Autodesk Inventor part; units mm, degrees
ref_plane "YZ Plane" through (0, 0, 0) normal (1, 0, 0) x (0, 1, 0)
ref_plane "XZ Plane" through (0, 0, 0) normal (0, 1, 0) x (-1, 0, 0)
ref_plane "XY Plane" through (0, 0, 0) normal (0, 0, 1) x (1, 0, 0)
sketch "Sketch1" plane through (0, 0, 0) normal (0, 1, 0) x (-1, 0, 0)
  line L0 (3.2, 1.8475) -> (3.2, -1.8475)
  line L1 (3.2, -1.8475) -> (0, -3.695)
  line L2 (0, -3.695) -> (-3.2, -1.8475)
  line L3 (-3.2, -1.8475) -> (-3.2, 1.8475)
  line L4 (-3.2, 1.8475) -> (0, 3.695)
  line L5 (0, 3.695) -> (3.2, 1.8475)
  point P0 (0, 0)
  point P1 (3.2, 0)
  point P2 (-3.2, 0)
  dimension "d0" = 6.4
  dimension "d1" = 120
  dimension "d2" = 6.4
extrude "Extrusion1" add sketch "Sketch1" along normal blind 11.96
sketch "Sketch2" plane through (0, 11.96, 0) normal (0, 1, 0) x (1, 0, 0)
  circle A0 centre (0, 0) radius 1.4224
  dimension "d5" = 2.8448
extrude "Extrusion2" add sketch "Sketch2" along normal blind 4.75
sketch "Sketch3" plane through (0, 0, 0) normal (0, -1, 0) x (1, 0, 0)
  circle A0 centre (0, 0) radius 1.4224
  dimension "d8" = 2.8448
extrude "Extrusion3" cut sketch "Sketch3" against normal blind 6.35
sketch "Sketch4" plane through (0, 0, 0) normal (0, -1, 0) x (1, 0, 0)
  circle A0 centre (0, 0) radius 1.4224
  line L0 (-3.2, -1.8475) -> (-3.2, 1.8475)
  line L1 (0, -3.695) -> (-3.2, -1.8475)
  line L2 (3.2, -1.8475) -> (0, -3.695)
  line L3 (3.2, 1.8475) -> (3.2, -1.8475)
  line L4 (0, 3.695) -> (3.2, 1.8475)
  line L5 (-3.2, 1.8475) -> (0, 3.695)
extrude "Extrusion4" add sketch "Sketch4" along normal blind 8.6233
sketch "Sketch5" plane through (0, 6.35, 0) normal (0, -1, 0) x (1, 0, 0)
  circle A0 centre (0, 0) radius 1.4224
extrude "Extrusion5" add sketch "Sketch5" along normal blind 8.6233
sketch "Sketch6" plane through (0, -8.6233, 0) normal (0, -1, 0) x (1, 0, 0)
  point P0 (0, 0)
sketch "Sketch7" plane through (0, -8.6233, 0) normal (0, -1, 0) x (1, 0, 0)
  line L0 (0, -3.695) -> (3.2, -1.8475)
  line L1 (3.2, -1.8475) -> (3.2, 1.8475)
  line L2 (3.2, 1.8475) -> (0, 3.695)
  line L3 (0, 3.695) -> (-3.2, 1.8475)
  line L4 (-3.2, 1.8475) -> (-3.2, -1.8475)
  line L5 (-3.2, -1.8475) -> (0, -3.695)
  circle A0 centre (0, 0) radius 1.4224
extrude "Extrusion6" cut sketch "Sketch7" against normal blind 10
sketch "Sketch8" plane through (0, -2.2733, 0) normal (0, -1, 0) x (1, 0, 0)
  circle A0 centre (0, 0) radius 1.4224
extrude "Extrusion7" cut sketch "Sketch8" against normal blind 9.817
sketch "Sketch9" plane through (0, 1.3767, 0) normal (0, -1, 0) x (1, 0, 0)
  line L0 (3.2, 1.8475) -> (3.2, -1.8475)
  line L1 (0, 3.695) -> (3.2, 1.8475)
  line L2 (-3.2, 1.8475) -> (0, 3.695)
  line L3 (-3.2, -1.8475) -> (-3.2, 1.8475)
  line L4 (0, -3.695) -> (-3.2, -1.8475)
  line L5 (3.2, -1.8475) -> (0, -3.695)
  circle A0 centre (0, 0) radius 1.4224
  circle A1 centre (0, 0) radius 1.4224
extrude "Extrusion8" cut sketch "Sketch9" against normal blind 1.058
sketch "Sketch10" plane through (0, 7.5437, 0) normal (0, -1, 0) x (1, 0, 0)
  circle A0 centre (0, 0) radius 1.4224
extrude "Extrusion9" cut sketch "Sketch10" against normal blind 1.058
properties part number "pcBOBAstandoff" material "Stainless Steel"
Geometry check sheet. Reference: the model listing, model coordinates, mm. A direction names the side the tool comes from. Coordinates: 2 decimals unless noted, no trailing zeros. Order: outer loops, then holes, each group sorted by start corner. A loop starts at its lowest first (then second) coordinate and runs counter-clockwise, first axis right, second up. Notation, with made-up numbers: (-9.75, -23.75) - (44.25, -23.75) arc R16 ccw to (44.25, -11.75) - close; hole circle Ø10 at (-4.5, -2.75). An arc over 180 degrees is marked (long way). Use one line per item in the form item = value.
1. Section check B-B (x = -1). Record the boundary of the cut face in (y, z).
Here are the results:
outline = (2.43, -3.12) - (11.96, -3.12) - (11.96, -1.01) - (16.71, -1.01) - (16.71, 1.01) - (11.96, 1.01) - (11.96, 3.12) - (2.43, 3.12) - (2.43, 1.01) - (8.6, 1.01) - (8.6, -1.01) - (2.43, -1.01) - close
2. Section check A-A (y = 7.5). Record the boundary of the cut face in (x, z) (1 decimal), then the cut area to 3 significant figures.
Here are the results:
outline = (-3.2, -1.8) - (0, -3.7) - (3.2, -1.8) - (3.2, 1.8) - (0, 3.7) - (-3.2, 1.8) - close; hole circle Ø2.8 at (0, 0)
area = 29.1 mm²
3. Draft check along X on faces 3 (the face through (0, 2.435, -2)), 4 (the face through (0, 8.602, 0)), 5 (the face through (-3.2, 7, 0)), 6 (the face through (-0.31, 5.48, -1.39)). Enter one of: pulls with the +X half, pulls with the -X half, needs draft (parallel to the pull), parting line crosses it, or undercut.
Here are the results:
face_3 = needs draft
face_4 = undercut
face_5 = pulls with the -X half
face_6 = undercut
4. Section check C-C (z = 1). Record the boundary of the cut face in (x, y), then the cut area to 3 significant figures.
Here are the results:
outline = (-3.2, 2.43) - (-1.01, 2.43) - (-1.01, 8.6) - (1.01, 8.6) - (1.01, 2.43) - (3.2, 2.43) - (3.2, 11.96) - (1.01, 11.96) - (1.01, 16.71) - (-1.01, 16.71) - (-1.01, 11.96) - (-3.2, 11.96) - close
area = 58.1 mm²
5. Access from +Z, -Z, +X, -X, +Y, -Y to the whole of each face (thin tool, end or side, straight path). Record for faces 1 (the face through (0, 11.96, -2)), 2 (the face through (1.62, 7.26, -2.76)).
Here are the results:
face_1 = +Y
face_2 = -Z, +X, +Y, -Y
6. Section check D-D (y = 9.75). Record the boundary of the cut face in (x, z) (1 decimal).
Here are the results:
outline = (-3.2, -1.8) - (0, -3.7) - (3.2, -1.8) - (3.2, 1.8) - (0, 3.7) - (-3.2, 1.8) - close
7. Gauge pin test, flat ends, axial feed: pin 1 (3 mm diameter, centred on x = 2, z = -1.5, fed in from +Y); pin 2 (0.9 mm diameter, centred on x = 0.5, z = -0.5, fed in from -Y); pin 3 (1 mm diameter, centred on x = 0.5, y = 13, fed in from +Z). Record the tip position at first contact, or that the pin passes through.
Here are the results:
pin_1 = 16.71
pin_2 = 8.6
pin_3 = 1.42
8. Scan lines: line 1 (Y direction, x = 0.5, z = -1); line 2 (Y direction, x = -1, z = 2.25); line 3 (X direction, y = 5.75, z = 1.25). Record each from-to range of solid material in increasing order.
Here are the results:
line_1 = 8.6 to 16.71
line_2 = 2.43 to 11.96
line_3 = -3.2 to -0.68, 0.68 to 3.2
